from build123d import *

# Parameters (mm, degrees)
F0_W     = 26.8387589604
F0_H     = 26.5057813376
F1_DEPTH = 17.78
F3_ANGLE = 180
F5_DEPTH = 12.7


with BuildPart() as f1:
    # F0 (on Top) → F1 (new body)
    with BuildSketch(Plane.XY):
        Rectangle(F0_W, F0_H)
    extrude(amount=F1_DEPTH)

    # F2 (on face) → F3 (revolve, cut)
    with BuildSketch(Plane.XY.offset(17.78)):
        with BuildLine():
            Line((-0.1599836294, 10.7320307857), (-0.010505857, -10.7332180251))
            ThreePointArc((-0.010505857, -10.7332180251), (10.7329629317, 0.0747412436), (-0.1599836294, 10.7320307857))
        make_face()
    revolve(axis=Axis((-0.0852447432, -0.0005936197, 17.78), (-0.0069635414, 0.9999757543, 0)), revolution_arc=F3_ANGLE, mode=Mode.SUBTRACT)

    # F4 (on face) → F5 (cut)
    with BuildSketch(Plane.XY.offset(17.78)):
        Polygon((2.006725641, 7.910721004), (-0.1403368457, 7.910721004), (-0.0334680846, -7.4358051643), (2.006725641, -7.4358051643), (2.006725641, -2.2563524544), (8.3371670917, -2.2563524544), (8.3371670917, 2.0598582923), (2.006725641, 2.0598582923), align=None)
        Polygon((-0.1403368457, 7.910721004), (-2.1176536102, 7.910721004), (-2.1176536102, 2.0598582923), (-8.6399270222, 2.0598582923), (-8.6399270222, -2.2563524544), (-2.1176536102, -2.2563524544), (-2.1176536102, -7.4358051643), (-0.0334680846, -7.4358051643), align=None)
    extrude(amount=-F5_DEPTH, mode=Mode.SUBTRACT)


solid = f1.part
Could you check a few things on this model? Use its own coordinates, in mm. A direction names the side the tool comes from. Coordinates: 2 decimals unless noted, no trailing zeros. Loops run counter-clockwise (first coordinate to the right, second up) from the corner with the lowest first, then second, coordinate; pieces in that order, holes last.
1. I need wall thicknesses on L1, parallel to X at y = -3.25, z = 6; L2, parallel to X at y = 4, z = 17; L3, parallel to Y at x = -2.25, z = 14.75. Which ranges of each line are inside material? Lowest first, please.
2. For P1, Ø1, axis at x = 4.5, y = 3, coming from the +Z side, with a flat end and sliding along its axis, tell me the tip position at first contact or that it passes through.
3. Imagine slicing it at A-A (z = 5.75). Please give me the cut outline in (x, y), and give its area (3 significant figures).
4. For faces 1 (the face through (0, 13.253, 9)), 2 (the face through (-2.118, -5, 7)), which set-ups out of +Z, -Z, +X, -X, +Y, -Y let a thin tool reach every point of the face, with its end or its side?
5. We'd pull the mould along X, two halves only. Please class faces 3 (the face through (0, 7.911, 8)), 4 (the face through (0, 12, 17.78)), 5 (the face through (13.419, 0, 9)): released by +X, released by -X, zero draft, split by the parting line, or undercut.
Computed values:
1. L1: x = -13.42 to -2.12, 2.01 to 13.42
1. L2: x = -13.42 to -10.1, 9.93 to 13.42
1. L3: y = -13.25 to -10.1, 10.1 to 13.25
2. P1: stops at z = 8.77
3. outline: (-13.42, -13.25) - (13.42, -13.25) - (13.42, 13.25) - (-13.42, 13.25) - close; hole (-8.64, -2.26) - (-2.12, -2.26) - (-2.12, -7.44) - (2.01, -7.44) - (2.01, -2.26) - (8.34, -2.26) - (8.34, 2.06) - (2.01, 2.06) - (2.01, 7.91) - (-2.12, 7.91) - (-2.12, 2.06) - (-8.64, 2.06) - close
3. area: 593 mm2
4. face 1: +Z, -Z, +X, -X, +Y
4. face 2: +Z
5. face 3: undercut
5. face 4: zero draft
5. face 5: released by +X
